Autodesk Inventor part; units mm, degrees
ref_plane "YZ Plane" through (0, 0, 0) normal (1, 0, 0) x (0, 1, 0)
ref_plane "XZ Plane" through (0, 0, 0) normal (0, 1, 0) x (-1, 0, 0)
ref_plane "XY Plane" through (0, 0, 0) normal (0, 0, 1) x (1, 0, 0)
ref_plane "Plano de trabajo1" through (188.0384, -192.9506, 83.6717) normal (0, 0, -1) x (-1, 0, 0)
sketch "Boceto2" plane through (188.0384, -192.9506, 83.6717) normal (0, 0, -1) x (-1, 0, 0)
  circle A0 centre (0, 0) radius 7.493
  circle A1 centre (0, 0) radius 3.175
  dimension "d6" = 14.986
  dimension "d7" = 6.35
sketch3d "Boceto 3D1"
  line L0 (260.8196, -237.5891, 75.5598) -> (249.4405, -237.6232, 75.5598)
  spline S0 degree 3 poles (188.0384, -192.9506, 83.6717) (188.0384, -192.9506, 58.2166) (223.9855, -237.6995, 75.5598) (249.4405, -237.6232, 75.5598) knots 0 0 0 0 7.63653 7.63653 7.63653 7.63653
  line L1 (188.0384, -192.9506, 83.6717) -> (188.0384, -192.9506, 102.9757)
  dimension "d4" = 1
  dimension "d5" = 1
sweep "Barrido1" add profiles "Boceto2" path "Boceto 3D1"
equation "\"d6\" = OD"
equation "\"d7\" = ID"
equation "\"ID\" = 6.35"
equation "\"OD\" = 14.986"
equation "\"L\" = PL"
equation "\"PL\" = 116.078"
equation "\"Size_Designation\" = 0.25"
equation "\"RPL\" = 117.475"
equation "\"OPL\" = 85.3948"
equation "\"ROPL\" = 85.725"
properties material "Caucho"
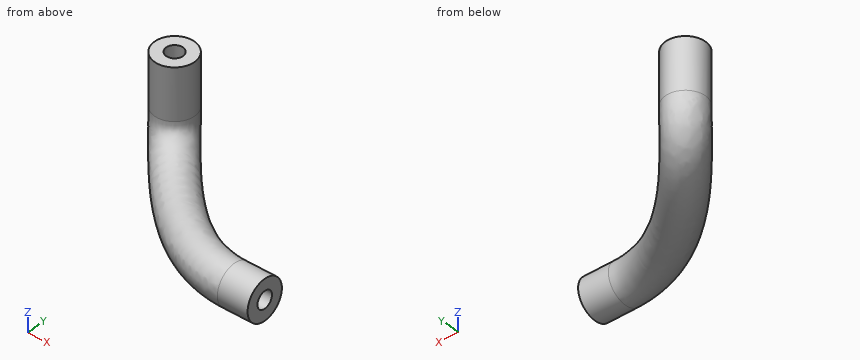
The model under review builds one solid part; all positions refer to its coordinate system, in mm. Coordinates: 2 decimals unless noted, no trailing zeros. Loops run counter-clockwise (first coordinate to the right, second up) from the corner with the lowest first, then second, coordinate; pieces in that order, holes last. Notation, with made-up numbers: (53, -11.75) -> (92, -11.75) arc R20 ccw to (92, 27.25) -> close; hole circle Ø10 at (-7, 29.25). An arc over 180 degrees is marked (long way). Use a Markdown table: item, result. Add a question column.
1. To check wall thickness, follow line 1 (Y direction, x = 246, z = 78); line 2 (Z direction, x = 225, y = -228.5); line 3 (Y direction, x = 189, z = 79). State the ranges of each line that lie inside material, in increasing order.
2. Add section B-B on z = 88.5. Write out the cut boundary in (x, y) (3 decimals).
3. Clearance check with flat-ended pins moving along their axes: pin 1 Ø1.5 at (x, z) = (197.5, 84) entering from +Y; pin 2 Ø4 at (y, z) = (-229.5, 69.5) entering from -X; pin 3 Ø8 at (x, z) = (235, 74) entering from +Y; pin 4 Ø12 at (y, z) = (-235.5, 81) entering from +X. State where each tip first meets the part, or that it passes through.
4. Add section A-A on z = 81.5. Give the number of separate pieces and of enclosed holes in the cut face, plus the area to 3 significant figures.
Returned:
| question | item | result |
|---|---|---|
| 1 | line 1 | y = -244.5 to -239.33, -235.46 to -230.26 |
| 1 | line 2 | z = 64.98 to 69.36, 75.74 to 80.12 |
| 1 | line 3 | y = -201.8 to -196.91, -190.34 to -185.9 |
| 2 | outline | circle Ø14.986 at (188.038, -192.951); hole circle Ø6.35 at (188.038, -192.951) |
| 3 | pin 1 | passes through |
| 3 | pin 2 | stops at x = 211.99 |
| 3 | pin 3 | stops at y = -223.08 |
| 3 | pin 4 | stops at x = 260.83 |
| 4 | separate pieces | 2 |
| 4 | enclosed holes | 1 |
| 4 | area | 371 mm² |
